Here's how the part is built. I have some questions about the finished solid (model axes, mm). A direction names the side the tool comes from. Round coordinates to 2 decimals unless told otherwise and drop trailing zeros. Order: outer loops, then holes, each group sorted by start corner. A loop starts at its lowest first (then second) coordinate and runs counter-clockwise, first axis right, second up. Notation, with made-up numbers: (8, -35.75) -> (22, -35.75) arc R29 cw to (22, -14.75) -> close; hole circle Ø5 at (1.25, -35). An arc over 180 degrees is marked (long way). One line per item, written item: value.
```python
from build123d import *

# Parameters (mm, degrees)
F1_DEPTH = 501.65
F2_R     = 2.38125
F3_DEPTH = 14.986
F4_R     = 2.38125
F5_DEPTH = 14.986
F6_R     = 2.54
F7_DEPTH = 31.751


with BuildPart() as f1:
    # F0 (on Right) → F1 (new body)
    with BuildSketch(Plane.YZ):
        Polygon((-39.572591, 38.912156), (-52.272591, 38.912156), (-52.272591, 26.212156), (-39.572591, 26.212156), (-39.572591, 16.687156), (58.852409, 16.687156), (71.552409, 7.162156), (71.552409, 11.911956), (58.852409, 21.436956), align=None)
    extrude(amount=-F1_DEPTH)

    # F2 (on face) → F3 (cut)
    with BuildSketch(Plane.YZ):
        with Locations((-26.872591, 26.212156)):
            Circle(F2_R)
        with Locations((-7.822591, 26.212156)):
            Circle(F2_R)
    extrude(amount=-F3_DEPTH, mode=Mode.SUBTRACT)

    # F4 (on face) → F5 (cut)
    with BuildSketch(Plane(origin=(-501.65, 0, 0), x_dir=(0, -1, 0), z_dir=(-1, 0, 0))):
        with Locations((26.872591, 26.212156)):
            Circle(F4_R)
        with Locations((7.822591, 26.212156)):
            Circle(F4_R)
    extrude(amount=-F5_DEPTH, mode=Mode.SUBTRACT)

    # F6 (on face) → F7 (cut, through all)
    with BuildSketch(Plane.XY.offset(38.912156)):
        with Locations((-450.85, -45.922591)):
            Circle(F6_R)
        with Locations((-333.375, -45.922591)):
            Circle(F6_R)
        with Locations((-168.275, -45.922591)):
            Circle(F6_R)
        with Locations((-50.8, -45.922591)):
            Circle(F6_R)
    extrude(amount=-F7_DEPTH, mode=Mode.SUBTRACT)


solid = f1.part
```
Q1. I want a section at C-C on y = 48.5. Write out the boundary of the cut face in (x, z) (3 decimals).
Answers:
outline: (-501.65, 16.687) -> (0, 16.687) -> (0, 23.275) -> (-501.65, 23.275) -> close
Q2. For P1, Ø12, axis at x = -170.5, z = 22.5, coming from the +Y side (3 decimals); P2, Ø10, axis at x = -268.5, y = -6, coming from the +Z side; P3, Ø1.5, axis at x = -235.5, z = 13.5, coming from the +Y side (3 decimals); P4, Ø8, axis at y = -17.5, z = 12, coming from the +X side, each with a flat end and sliding along its axis, tell me the tip position at first contact or that it passes through.
Answers:
P1: y = 65.435
P2: z = 33.84
P3: y = 70.435
P4: through
Q3. I want a section at A-A on x = -228.5. Write out the boundary of the cut face in (y, z).
Answers:
outline: (-52.27, 26.21) -> (-39.57, 26.21) -> (-39.57, 16.69) -> (58.85, 16.69) -> (71.55, 7.16) -> (71.55, 11.91) -> (58.85, 21.44) -> (-39.57, 38.91) -> (-52.27, 38.91) -> close
Q4. I want a section at B-B on y = 25. Write out the boundary of the cut face in (x, z).
Answers:
outline: (-501.65, 16.69) -> (0, 16.69) -> (0, 27.45) -> (-501.65, 27.45) -> close
Q5. I need wall thicknesses on line 1 along Z through (x, y) = (-173, 18.5); line 2 along Z through (x, y) = (-81.5, -23.5); line 3 along Y through (x, z) = (-168.5, 12.5). Which ranges of each line are inside material? Lowest first, please.
Answers:
line 1: 16.69 to 28.6
line 2: 16.69 to 36.06
line 3: 64.44 to 70.77
Q6. Which directions (+Z, -Z, +X, -X, +Y, -Y) give clear straight access to the entire face, cutting with the end or side of a thin tool? Please do faces 1 (the face through (-247, -46, 38.912)), 2 (the face through (-247, 9, 16.687)).
Answers:
face 1: +Z, +X, -X, +Y, -Y
face 2: -Z, +X, -X, -Y
